from build123d import *

# Parameters (mm, degrees)
SKETCH1_W           = 14.5
SKETCH1_H           = 24.5
SKETCH1_R           = 0.85
BOSS_EXTRUDE1_DEPTH = 7
CHAMFER1_SIZE       = 1
SKETCH2_R           = 1.75
CUT_EXTRUDE1_DEPTH  = 22.836036728
SKETCH3_R           = 3
CUT_EXTRUDE2_DEPTH  = 3


with BuildPart() as part:
    # Sketch1 → Boss-Extrude1 (new body)
    with BuildSketch(Plane(origin=(0, 0, 0), x_dir=(0, 0, -1), z_dir=(1, 0, 0))):
        with Locations((0.75, -2.5)):
            Rectangle(SKETCH1_W, SKETCH1_H)
        with Locations((0, 4.75)):
            Circle(SKETCH1_R, mode=Mode.SUBTRACT)
        with Locations((0, -4.75)):
            Circle(SKETCH1_R, mode=Mode.SUBTRACT)
    extrude(amount=BOSS_EXTRUDE1_DEPTH)

    # Chamfer1
    chamfer1_edges = [part.edges().sort_by_distance(p)[0] for p in [
        (7, -2.5, -8),
        (0, -2.5, -8),
    ]]
    chamfer(chamfer1_edges, length=CHAMFER1_SIZE)

    # Sketch2 → Cut-Extrude1 (cut, through all)
    with BuildSketch(Plane.XY.offset(6.5)):
        with Locations((3.5, 0.25)):
            Circle(SKETCH2_R)
        with Locations((3.5, -9.75)):
            Circle(SKETCH2_R)
    extrude(amount=-CUT_EXTRUDE1_DEPTH, mode=Mode.SUBTRACT)

    # Sketch3 → Cut-Extrude2 (cut)
    with BuildSketch(Plane.XY.offset(6.5)):
        with Locations((3.5, 0.25)):
            Circle(SKETCH3_R)
        with Locations((3.5, -9.75)):
            Circle(SKETCH3_R)
    extrude(amount=-CUT_EXTRUDE2_DEPTH, mode=Mode.SUBTRACT)


solid = part.part
Design review of the part built by this model. Coordinates are the model's own, in mm. A direction names the side the tool comes from. Round coordinates to 2 decimals unless told otherwise and drop trailing zeros. Loops run counter-clockwise (first coordinate to the right, second up) from the corner with the lowest first, then second, coordinate; pieces in that order, holes last. Notation, with made-up numbers: (31, 16.25) -> (77, 16.25) arc R15 ccw to (77, 45.25) -> close; hole circle Ø3 at (-3.5, 51.25). An arc over 180 degrees is marked (long way). Use one line per item in the form item = value. Start each with the question number.
Q1. For pin 1 Ø1.5 at (y, z) = (-4.75, 0) entering from +X; pin 2 Ø1 at (x, y) = (1.5, 1) entering from +Z, all flat-tipped, find the tip position at first contact; note any pin that passes through.
Q2. Draft analysis for pull direction Z (two halves, no side actions). For faces 3 (the face through (5, -1, 3.5)), 4 (the face through (0.5, -2.7, -7.5)), 5 (the face through (3.45, -5.58, 0.18)), state which applies: +Z half, -Z half, draft (parallel to the pull), parting line (faces both ways), or undercut.
Q3. Wall thickness on line 1 along Y through (x, z) = (4.75, 0); line 2 along Y through (x, z) = (3.5, 0.25); line 3 along Y through (x, z) = (4.25, 1.75): over which ranges is each line inside the solid? List them lowest first. Write a range as [from, to].
Q4. We need section A-A on x = 3.5. Give the boundary of the cut face in (y, z), then the cut area to 3 significant figures.
Q5. We need section C-C on z = -3.75. Give the boundary of the cut face in (x, y).
Q6. We need section D-D on y = -1.25. Give the boundary of the cut face in (x, z).
Q7. We need section B-B on y = -9.75. Give the boundary of the cut face in (x, z), then the cut area to 4 significant figures.
Q8. Machinability: for faces 1 (the face through (0, -2, 0)), 2 (the face through (5, -11, 3.5)), which of the approach directions +Z, -Z, +X, -X, +Y, -Y give a long, thin tool a straight path to every point of the face, cutting with its end or side? Answer none if there is none.
Calculated:
q1.pin_1 = through
q1.pin_2 = 3.5
q2.face_3 = +Z half
q2.face_4 = -Z half
q2.face_5 = undercut
q3.line_1 = [-14.75, -10.97], [-8.53, -5.6], [-3.9, -0.97], [1.47, 3.9], [5.6, 9.75]
q3.line_2 = [-14.75, -11.5], [-8, -5.56], [-3.94, -1.5], [2, 3.94], [5.56, 9.75]
q3.line_3 = [-14.75, -11.33], [-8.17, -1.33], [1.83, 9.75]
q4.outline = (-14.75, -8) -> (-11.5, -8) -> (-11.5, 3.5) -> (-12.75, 3.5) -> (-12.75, 6.5) -> (-14.75, 6.5) -> close; (-8, -8) -> (-1.5, -8) -> (-1.5, 3.5) -> (-2.75, 3.5) -> (-2.75, 6.5) -> (-6.75, 6.5) -> (-6.75, 3.5) -> (-8, 3.5) -> close; (2, -8) -> (9.75, -8) -> (9.75, 6.5) -> (3.25, 6.5) -> (3.25, 3.5) -> (2, 3.5) -> close; hole circle Ø1.7 at (-4.75, 0); hole circle Ø1.7 at (4.75, 0)
q4.area = 234 mm²
q5.outline = (0, -14.75) -> (7, -14.75) -> (7, 9.75) -> (0, 9.75) -> close; hole circle Ø3.5 at (3.5, -9.75); hole circle Ø3.5 at (3.5, 0.25)
q6.outline = (0, -7) -> (1, -8) -> (2.6, -8) -> (2.6, 3.5) -> (0.9, 3.5) -> (0.9, 6.5) -> (0, 6.5) -> close; (4.4, -8) -> (6, -8) -> (7, -7) -> (7, 6.5) -> (6.1, 6.5) -> (6.1, 3.5) -> (4.4, 3.5) -> close
q7.outline = (0, -7) -> (1, -8) -> (1.75, -8) -> (1.75, 3.5) -> (0.5, 3.5) -> (0.5, 6.5) -> (0, 6.5) -> close; (5.25, -8) -> (6, -8) -> (7, -7) -> (7, 6.5) -> (6.5, 6.5) -> (6.5, 3.5) -> (5.25, 3.5) -> close
q7.area = 42.25 mm²
q8.face_1 = +Z, -Z, -X, +Y, -Y
q8.face_2 = +Z
